Model file for the job. Use its own axes, mm. A direction names the side the tool comes from. Give positions to 0.01 mm unless a question says otherwise; leave off trailing zeros. Loops run counter-clockwise (first coordinate to the right, second up) from the corner with the lowest first, then second, coordinate; pieces in that order, holes last. Notation, with made-up numbers: (72.5, 33.5) -> (114.5, 33.5) arc R6 cw to (114.5, 38.5) -> close; hole circle Ø7 at (2, -18.5). An arc over 180 degrees is marked (long way). Use CSV: the item, a comma, the result in double quotes. Start each with the question number.
(1) Cut at C-C on x = 64. Write the cut outline in (y, z).
(2) Drill centre lines: probe 1 along Y at (x, z) = (86.5, 1.2); probe 2 along X at (y, z) = (-42, -104.5); probe 3 along Z at (x, y) = (-117, 58). Where is each one in solid material? Low to high.
(3) Cut at B-B on z = -215. Write the cut outline in (x, y), then the cut area to 3 significant figures.
(4) Pull direction Z, two halves, no side cores. Call faces 1 (the cylindrical face through (81.881, -5.585, 2.465)), 2 (the flat face through (-1, 1, -1)), 3 (the cylindrical face through (-157.37, 81.69, -186.13)): pulls with the +Z half, pulls with the -Z half, needs draft (parallel to the pull), parting line crosses it, or undercut.
(5) Cut at A-A on y = -18. Write the cut outline in (x, z), then the cut area to 3 significant figures.
(6) Flat gauge pins, fed straight in: pin 1 (3 mm diameter, centred on y = 78.5, z = -292.5, fed in from -X); pin 2 (12 mm diameter, centred on x = 7.5, y = -4, fed in from -Z); pin 3 (9 mm diameter, centred on y = 78.45, z = -402.61, fed in from +X). Where does each tip first touch, or does it go through?
(7) 3-axis set-ups, long thin cutter, end or side, ignore diameter. For faces 4 (the flat face through (-147.5, -2, -237)), 5 (the cylindrical face through (-157.374, 83.207, -73.209)), 6 (the flat face through (-157, 86.5, -230)): which of +Z, -Z, +X, -X, +Y, -Y reach the whole face in a straight line?
from build123d import *

# Parameters (mm, degrees)
SKETCH1_W                    = 297
SKETCH1_H                    = 175
BASE_FLANGE1_DEPTH           = 1
EDGE_FLANGE1_STRIP_W         = 5.4732
EDGE_FLANGE1_STRIP_H         = 1
EDGE_FLANGE1_STRIP_CUT_DEPTH = 175
EDGE_FLANGE1_DEPTH           = 175
EDGE_FLANGE2_STRIP_W         = 5.4732
EDGE_FLANGE2_STRIP_H         = 1
EDGE_FLANGE2_STRIP_CUT_DEPTH = 463.2634
EDGE_FLANGE2_DEPTH           = 463.2634
SKETCH17_R                   = 4.794
SKETCH17_R_2                 = 2.794
BOSS_EXTRUDE1_DEPTH          = 18
SKETCH21_R                   = 5
SKETCH21_R_2                 = 3
BOSS_EXTRUDE2_DEPTH          = 5


# Sheet-metal steps are written as plain solids
with BuildPart() as part:
    # Sketch1 → Base-Flange1 (new body)
    with BuildSketch(Plane.XY):
        Rectangle(SKETCH1_W, SKETCH1_H)
    extrude(amount=-BASE_FLANGE1_DEPTH)

    # Edge-Flange1 strip (across the edge) → Edge-Flange1 strip cut (cut)
    with BuildSketch(Plane(origin=(-148.5, -87.5, -1), x_dir=(1, 0, 0), z_dir=(0, 1, 0))):
        with Locations((-1, -0.5)):
            Rectangle(EDGE_FLANGE1_STRIP_W, EDGE_FLANGE1_STRIP_H)
    extrude(amount=EDGE_FLANGE1_STRIP_CUT_DEPTH, mode=Mode.SUBTRACT)

    # Edge-Flange1 section (across the edge) → Edge-Flange1 (add)
    with BuildSketch(Plane(origin=(-148.5, -87.5, -1), x_dir=(1, 0, 0), z_dir=(0, 1, 0))):
        with BuildLine():
            Line((0, 0.7366), (0, 464))
            Line((0, 464), (1, 464))
            Line((1, 464), (1, 0.7366))
            ThreePointArc((1, 0.7366), (1.215745145, 0.215745145), (1.7366, 0))
            Line((1.7366, 0), (1.7366, -1))
            ThreePointArc((1.7366, -1), (0.508638364, -0.491361636), (0, 0.7366))
        make_face()
    extrude(amount=EDGE_FLANGE1_DEPTH)

    # Edge-Flange2 strip (across the edge) → Edge-Flange2 strip cut (cut)
    with BuildSketch(Plane(origin=(-148.5, 87.5, -1.7366), x_dir=(0, -1, 0), z_dir=(0, 0, -1))):
        with Locations((-1, -0.5)):
            Rectangle(EDGE_FLANGE2_STRIP_W, EDGE_FLANGE2_STRIP_H)
    extrude(amount=EDGE_FLANGE2_STRIP_CUT_DEPTH, mode=Mode.SUBTRACT)

    # Edge-Flange2 section (across the edge) → Edge-Flange2 (add)
    with BuildSketch(Plane(origin=(-148.5, 87.5, -1.7366), x_dir=(0, -1, 0), z_dir=(0, 0, -1))):
        with BuildLine():
            Line((0, 0.7366), (0, 17))
            Line((0, 17), (1, 17))
            Line((1, 17), (1, 0.7366))
            ThreePointArc((1, 0.7366), (1.215745145, 0.215745145), (1.7366, 0))
            Line((1.7366, 0), (1.7366, -1))
            ThreePointArc((1.7366, -1), (0.508638364, -0.491361636), (0, 0.7366))
        make_face()
    extrude(amount=EDGE_FLANGE2_DEPTH)

    # Sketch17 → Boss-Extrude1 (add)
    # profile 1 of 4: a face of its own
    with BuildSketch(Plane.ZY.offset(148.5)):
        with Locations((-72.584668807, 78.453866984)):
            Circle(SKETCH17_R)
        with Locations((-72.584668807, 78.453866984)):
            Circle(SKETCH17_R_2, mode=Mode.SUBTRACT)
    # profile 2 of 4: a face of its own
    with BuildSketch(Plane.ZY.offset(148.5)):
        with Locations((-182.592068807, 78.453866984)):
            Circle(SKETCH17_R)
        with Locations((-182.592068807, 78.453866984)):
            Circle(SKETCH17_R_2, mode=Mode.SUBTRACT)
    # profile 3 of 4: a face of its own
    with BuildSketch(Plane.ZY.offset(148.5)):
        with Locations((-292.599468807, 78.453866984)):
            Circle(SKETCH17_R)
        with Locations((-292.599468807, 78.453866984)):
            Circle(SKETCH17_R_2, mode=Mode.SUBTRACT)
    # profile 4 of 4: a face of its own
    with BuildSketch(Plane.ZY.offset(148.5)):
        with Locations((-402.606868807, 78.453866984)):
            Circle(SKETCH17_R)
        with Locations((-402.606868807, 78.453866984)):
            Circle(SKETCH17_R_2, mode=Mode.SUBTRACT)
    extrude(amount=BOSS_EXTRUDE1_DEPTH)

    # Sketch21 → Boss-Extrude2 (add)
    # profile 1 of 2: a face of its own
    with BuildSketch(Plane.XY):
        with Locations(Location((86.5, 52.5, 0), (0, 0, 180))):
            Circle(SKETCH21_R)
        with Locations((86.5, 52.5)):
            Circle(SKETCH21_R_2, mode=Mode.SUBTRACT)
    # profile 2 of 2: a face of its own
    with BuildSketch(Plane.XY):
        with Locations(Location((86.5, -7.5, 0), (0, 0, 180))):
            Circle(SKETCH21_R)
        with Locations((86.5, -7.5)):
            Circle(SKETCH21_R_2, mode=Mode.SUBTRACT)
    extrude(amount=BOSS_EXTRUDE2_DEPTH)


solid = part.part
Check result:
1,outline,"(-87.5, -1) -> (87.5, -1) -> (87.5, 0) -> (-87.5, 0) -> close"
2,probe 1,"-12.5 to -10.5, -4.5 to -2.5, 47.5 to 49.5, 55.5 to 57.5"
2,probe 2,"-148.5 to -147.5"
2,probe 3,"-1 to 0"
3,outline,"(-165.5, 86.5) -> (-149.24, 86.5) arc R0.74 cw to (-148.5, 85.76) -> (-148.5, -87.5) -> (-147.5, -87.5) -> (-147.5, 85.76) arc R1.74 ccw to (-149.24, 87.5) -> (-165.5, 87.5) -> close"
3,area,"191 mm²"
4,face 1,"needs draft"
4,face 2,"pulls with the -Z half"
4,face 3,"undercut"
5,outline,"(-148.5, -465) -> (-147.5, -465) -> (-147.5, -1.74) arc R0.74 cw to (-146.76, -1) -> (148.5, -1) -> (148.5, 0) -> (-146.76, 0) arc R1.74 ccw to (-148.5, -1.74) -> close"
5,area,"760 mm²"
6,pin 1,"x = -148.5"
6,pin 2,"z = -1"
6,pin 3,"x = -147.5"
7,face 4,"-Z, +X, +Y, -Y"
7,face 5,"-X"
7,face 6,"+Z, -Z, -X"
